Job drawing, mm, ordinate dimensions from the low corner. One solid piece. Round coordinates to 2 decimals unless told otherwise and drop trailing zeros. Write each loop counter-clockwise with the first axis right and the second up, starting at its lowest first coordinate (ties: lowest second). Pieces come first, ordered by that corner, then holes.
1) Flat gauge pins, fed straight in: pin 1 (2 mm diameter, centred on x = 46, z = 114, fed in from -Y); pin 2 (8 mm diameter, centred on x = 110.5, y = 77.5, fed in from +Z); pin 3 (4 mm diameter, centred on x = 91, y = 59, fed in from +Z). Where does each tip first touch, or does it go through?
2) Drill centre lines: L1, parallel to Z at x = 78.5, y = 135; L2, parallel to Y at x = 16, z = 114; L3, parallel to Z at x = 81, y = 146.5. Where is each one in solid material? Low to high.
3) Saw through at B-B on y = 140. Write the cut outline in (x, z), and give its area (3 significant figures).
4) Saw through at C-C on z = 93.5. Write the cut outline in (x, y), and give its area (3 significant figures).
5) Saw through at A-A on x = 44.5. Write the cut outline in (y, z).
6) Saw through at D-D on z = 112. Write the cut outline in (x, y).
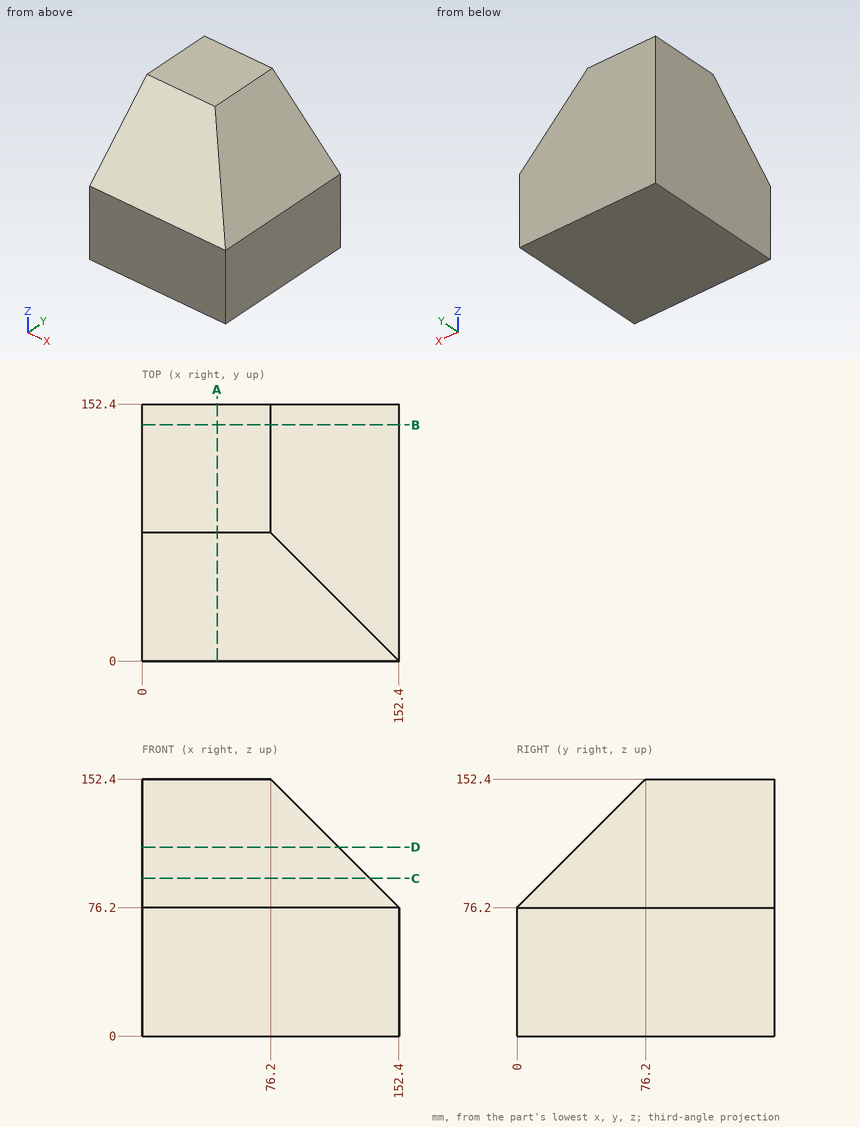
Completed:
1. pin 1: stops at y = 36.8
1. pin 2: stops at z = 122.1
1. pin 3: stops at z = 137.2
2. L1: z = 0 to 150.1
2. L2: y = 37.8 to 152.4
2. L3: z = 0 to 147.6
3. outline: (0, 0) - (152.4, 0) - (152.4, 76.2) - (76.2, 152.4) - (0, 152.4) - close
3. area: 20,300 mm2
4. outline: (0, 17.3) - (135.1, 17.3) - (135.1, 152.4) - (0, 152.4) - close
4. area: 18,300 mm2
5. outline: (0, 0) - (152.4, 0) - (152.4, 152.4) - (76.2, 152.4) - (0, 76.2) - close
6. outline: (0, 35.8) - (116.6, 35.8) - (116.6, 152.4) - (0, 152.4) - close
